Verification items for the finished model (mm, model axes). Round coordinates to 2 decimals unless told otherwise and drop trailing zeros. Write each loop counter-clockwise with the first axis right and the second up, starting at its lowest first coordinate (ties: lowest second). Pieces come first, ordered by that corner, then holes. Notation, with made-up numbers: M 41.5,76 L 77.5,76 A29 cw 77.5,113 Z; hole C 15.5,53.25 d5. An arc over 180 degrees is marked long. One line per item, written item: value. Start each with the question number.
from build123d import *

# Parameters (mm, degrees)
F0_W     = 233.8
F0_H     = 233.8
F1_DEPTH = 3
F2_R     = 12.5
F3_DEPTH = 3.001
F4_SIZE  = 3


with BuildPart() as f1:
    # F0 (on Top) → F1 (new body)
    with BuildSketch(Plane.XY):
        Rectangle(F0_W, F0_H)
    extrude(amount=F1_DEPTH)

    # F2 (on face) → F3 (cut, through all)
    with BuildSketch(Plane.XY.offset(3)):
        with Locations((-60, 60)):
            Circle(F2_R)
        with Locations((-60, -60)):
            Circle(F2_R)
        with Locations((60, -60)):
            Circle(F2_R)
        with Locations((60, 60)):
            Circle(F2_R)
    extrude(amount=-F3_DEPTH, mode=Mode.SUBTRACT)

    # F4
    f4_edges = [f1.edges().sort_by_distance(p)[0] for p in [
        (116.9, 116.9, 1.5),
        (-116.9, 116.9, 1.5),
        (116.9, -116.9, 1.5),
        (-116.9, -116.9, 1.5),
    ]]
    chamfer(f4_edges, length=F4_SIZE)


solid = f1.part
1) Cross-section at C-C (z = 0.8). Record the boundary of the cut face in (x, y), then the cut area to 3 significant figures.
2) Mould release check, pull along Y, two halves, no side actions. Record for faces 1 (the cylindrical face through (-61.627, 72.394, 1.521)), 2 (the flat face through (-2, 2, 3)), 3 (the cylindrical face through (50.79, -51.55, 1.52)): pulls with the +Y half, pulls with the -Y half, needs draft (parallel to the pull), parting line crosses it, or undercut.
3) Cross-section at A-A (y = -60). Record the boundary of the cut face in (x, z).
4) Thickness scan on line 1 (Y direction, x = 60, z = 1); line 2 (Y direction, x = 69.5, z = 2.15). Record the ranges inside material, lowest first.
Results below:
1. outline: M -116.9,-113.9 L -113.9,-116.9 L 113.9,-116.9 L 116.9,-113.9 L 116.9,113.9 L 113.9,116.9 L -113.9,116.9 L -116.9,113.9 Z; hole C -60,-60 d25; hole C -60,60 d25; hole C 60,-60 d25; hole C 60,60 d25
1. area: 52,700 mm²
2. face 1: undercut
2. face 2: needs draft
2. face 3: undercut
3. outline: M -116.9,0 L -72.5,0 L -72.5,3 L -116.9,3 Z; M -47.5,0 L 47.5,0 L 47.5,3 L -47.5,3 Z; M 72.5,0 L 116.9,0 L 116.9,3 L 72.5,3 Z
4. line 1: y = -116.9 to -72.5, -47.5 to 47.5, 72.5 to 116.9
4. line 2: y = -116.9 to -68.12, -51.88 to 51.88, 68.12 to 116.9
